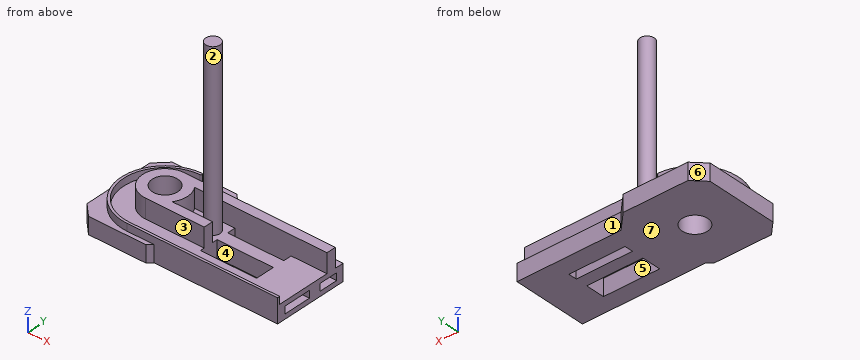
from build123d import *

# Parameters (mm, degrees)
SKETCH1_R               = 5.35
BOSS_EXTRUDE2_DEPTH     = 7
BOSS_EXTRUDE3_START     = 8
SKETCH3_R               = 5.35
BOSS_EXTRUDE3_DEPTH     = 8
BOSS_EXTRUDE4_DEPTH     = 3
CHAMFER1_SIZE           = 10
CHAMFER2_SIZE           = 5
CUT_EXTRUDE1_DEPTH      = 67.560662475
CUT_EXTRUDE1_DEPTH_BACK = 67.560662475
SKETCH5_W               = 23.474956737
SKETCH5_H               = 3.5
SKETCH5_H_2             = 8
CHAMFER3_SIZE           = 7
SKETCH6_W               = 3
SKETCH6_H               = 8.094956055
SKETCH6_H_2             = 11.655043945
CUT_EXTRUDE2_DEPTH      = 5
CUT_EXTRUDE3_REACH      = 87.249
SKETCH7_W               = 8
SKETCH7_H               = 4
SKETCH8_R               = 3
BOSS_EXTRUDE5_DEPTH     = 72
FILLET1_R               = 0.5


# Some blends are built 0.0001 mm under size
with BuildPart() as part:
    # Sketch1 → Boss-Extrude2 (new body)
    with BuildSketch(Plane.XY):
        Polygon((-19.503784034, -20), (19.503784034, -20), (19.503784034, -18.25), (62.978740771, -18.25), (62.978740771, 13), (19.503784034, 13), (19.503784034, 20), (-19.503784034, 20), align=None)
        Circle(SKETCH1_R, mode=Mode.SUBTRACT)
    extrude(amount=-BOSS_EXTRUDE2_DEPTH)

    # Sketch3 → Boss-Extrude3 (add)
    with BuildSketch(Plane.XY.offset(BOSS_EXTRUDE3_START)):
        with BuildLine():
            Line((7.668115805, 5.35), (62.978740771, 5.35))
            Line((62.978740771, 5.35), (62.978740771, 9.35))
            Line((62.978740771, 9.35), (0, 9.35))
            ThreePointArc((0, 9.35), (-9.35, 0), (0, -9.35))
            Line((0, -9.35), (62.978740771, -9.35))
            Line((62.978740771, -9.35), (62.978740771, -5.35))
            Line((62.978740771, -5.35), (7.668115805, -5.35))
            ThreePointArc((7.668115805, -5.35), (9.35, 0), (7.668115805, 5.35))
        make_face()
        Circle(SKETCH3_R, mode=Mode.SUBTRACT)
    extrude(amount=-BOSS_EXTRUDE3_DEPTH)

    # Sketch4 → Boss-Extrude4 (add)
    with BuildSketch(Plane.XY):
        with BuildLine():
            Line((0, -18.25), (62.978740771, -18.25))
            Line((62.978740771, -18.25), (62.978740771, -17.25))
            Line((62.978740771, -17.25), (8.306623863, -17.25))
            Line((8.306623863, -17.25), (0, -17.25))
            ThreePointArc((0, -17.25), (-17.25, 0), (0, 17.25))
            Line((0, 17.25), (0, 18.25))
            ThreePointArc((0, 18.25), (-18.25, 0), (0, -18.25))
        make_face()
    extrude(amount=BOSS_EXTRUDE4_DEPTH)

    # Chamfer1
    # the kernel refuses this chamfer: 10 mm, written as the material it takes off along each edge
    with BuildSketch(Plane(origin=(19.503784034, -20, 25.71682988), x_dir=(-0.9996219169112968, -0.027495876610586317, 0), z_dir=(0, 0, -1))) as chamfer1_piece_1_section:
        Polygon((CHAMFER1_SIZE * 0.999621916911, CHAMFER1_SIZE * 0.0274958766106), (-CHAMFER1_SIZE * 0.0274958766106, CHAMFER1_SIZE * 0.999621916911), (0, 0), align=None)
    chamfer1_piece_1 = extrude(amount=58.433659759, mode=Mode.PRIVATE)
    chamfer1_piece_1 = split(chamfer1_piece_1, bisect_by=Plane(origin=(14.814200223, -18.25, -3.5), z_dir=(0, -1, 0)), keep=Keep.TOP, mode=Mode.PRIVATE)
    add(chamfer1_piece_1, mode=Mode.SUBTRACT)

    # Chamfer2
    chamfer2_edges = [part.edges().sort_by_distance(p)[0] for p in [
        (-19.503784034, -20, -3.5),
        (-19.503784034, 20, -3.5),
    ]]
    chamfer(chamfer2_edges, length=CHAMFER2_SIZE)

    # Sketch5 → Cut-Extrude1 (cut, two sides: drawn at the far end of the back side and taken through both)
    with BuildSketch(Plane.XY.offset(-CUT_EXTRUDE1_DEPTH_BACK)):
        with Locations((36.241262403, 3.6)):
            Rectangle(SKETCH5_W, SKETCH5_H)
        with Locations((36.241262403, -7.15)):
            Rectangle(SKETCH5_W, SKETCH5_H_2)
    extrude(amount=CUT_EXTRUDE1_DEPTH + CUT_EXTRUDE1_DEPTH_BACK, mode=Mode.SUBTRACT)

    # Chamfer3
    chamfer3_edges = [part.edges().sort_by_distance(p)[0] for p in [
        (19.503784034, 20, -3.5),
    ]]
    chamfer(chamfer3_edges, length=CHAMFER3_SIZE - 0.0001)  # a hair under: the kernel refuses the full size

    # Sketch6 → Cut-Extrude2 (cut)
    with BuildSketch(Plane(origin=(62.978740771, 0, 0), x_dir=(0, 0, -1), z_dir=(1, 0, 0))):
        with Locations((3.5, 5.952521972)):
            Rectangle(SKETCH6_W, SKETCH6_H)
        with Locations((3.5, -8.922478028)):
            Rectangle(SKETCH6_W, SKETCH6_H_2)
    extrude(amount=-CUT_EXTRUDE2_DEPTH, mode=Mode.SUBTRACT)

    # Sketch7 → Cut-Extrude3 (cut, up to next)
    with BuildSketch(Plane(origin=(62.978740771, 0, 0), x_dir=(0, 0, -1), z_dir=(1, 0, 0)), mode=Mode.PRIVATE) as cut_extrude3_sk1:
        with Locations((-4, -7.35)):
            Rectangle(SKETCH7_W, SKETCH7_H)
    cut_extrude3_tool1 = extrude(cut_extrude3_sk1.sketch, amount=-CUT_EXTRUDE3_REACH, mode=Mode.PRIVATE) & part.part
    add(cut_extrude3_tool1.solids().sort_by_distance((62.978741, -7.35, 4))[0], mode=Mode.SUBTRACT)

    # Sketch8 → Boss-Extrude5 (add)
    with BuildSketch(Plane.XY):
        with Locations((20.003784034, 0)):
            Circle(SKETCH8_R)
    extrude(amount=BOSS_EXTRUDE5_DEPTH)

    # Fillet1
    fillet1_edges = [part.edges().sort_by_distance(p)[0] for p in [
        (0, 18.25, 1.5),
        (0, 17.25, 1.5),
    ]]
    fillet(fillet1_edges, radius=FILLET1_R - 0.0001)  # a hair under: the kernel refuses the full size


solid = part.part
For this review, take the finished solid that the model builds, in its own axes (mm). Face numbers are marked on the shaded views. A direction names the side the tool comes from. Give positions to 0.01 mm unless a question says otherwise; leave off trailing zeros. Loops run counter-clockwise (first coordinate to the right, second up) from the corner with the lowest first, then second, coordinate; pieces in that order, holes last.
Item 1: Tool access review of the marked faces 1, 2, 3 and 4: name each direction out of +Z, -Z, +X, -X, +Y, -Y from which nothing blocks a thin tool from reaching the whole face with its end or side.
Item 2: Take a section at B-B, the plane x = -3.5. State the section outline as (y, z) points, and give its area (3 significant figures).
Item 3: For line 1 along Y through (x, z) = (0, -1); line 2 along Z through (x, y) = (56, 8); line 3 along Z through (x, y) = (8, 11), list the stretches that pass through material, from the lowest coordinate up.
Item 4: Take a section at C-C, the plane x = 27. State the section outline as (y, z) points.
Item 5: Take a section at A-A, the plane y = 0. State the section outline as (x, z) points.
Item 6: Draft analysis for pull direction X (two halves, no side actions). For the marked faces 5, 6 and 7, state which applies: +X half, -X half, draft (parallel to the pull), parting line (faces both ways), or undercut.
Item 7: Take a section at D-D, the plane x = 51. State the section outline as (y, z) points, and give its area (3 significant figures).
Item 8: Insertion check: pin 1 (5.5 mm diameter, centred on x = 38.5, y = -1.5, fed in from +Z); pin 2 (17 mm diameter, centred on x = 0, y = 0, fed in from +Z); pin 3 (3.5 mm diameter, centred on x = 60, z = -3, fed in from -Y). Each pin has a flat end and moves straight along its axis. Give the tip position at first contact, or say it passes through.
Calculated:
1. face 1: +Z, -Z, +X, +Y
1. face 2: +Z
1. face 3: +Z, +X
1. face 4: +Z, -Z
2. outline: (-20, -7) - (-4.05, -7) - (-4.05, 8) - (-8.67, 8) - (-8.67, 0) - (-16.89, 0) - (-16.89, 3) - (-17.91, 3) - (-17.91, 0) - (-20, 0) - close; (4.05, -7) - (20, -7) - (20, 0) - (17.91, 0) - (17.91, 3) - (16.89, 3) - (16.89, 0) - (8.67, 0) - (8.67, 8) - (4.05, 8) - close
2. area: 303 mm2
3. line 1: y = -20 to -5.35, 5.35 to 20
3. line 2: z = -7 to 8
3. line 3: z = -7 to 0
4. outline: (-18.25, -7) - (-11.15, -7) - (-11.15, 0) - (-17.25, 0) - (-17.25, 3) - (-18.25, 3) - close; (-3.15, -7) - (1.85, -7) - (1.85, 0) - (-3.15, 0) - close; (5.35, -7) - (13, -7) - (13, 0) - (9.35, 0) - (9.35, 8) - (5.35, 8) - close
5. outline: (-19.5, -7) - (-5.35, -7) - (-5.35, 8) - (-9.35, 8) - (-9.35, 0) - (-17.25, 0) - (-17.25, 3) - (-18.25, 3) - (-18.25, 0) - (-19.5, 0) - close; (5.35, -7) - (62.98, -7) - (62.98, 0) - (23, 0) - (23, 72) - (17, 72) - (17, 0) - (9.35, 0) - (9.35, 8) - (5.35, 8) - close
6. face 5: undercut
6. face 6: -X half
6. face 7: draft
7. outline: (-18.25, -7) - (13, -7) - (13, 0) - (9.35, 0) - (9.35, 8) - (5.35, 8) - (5.35, 0) - (-17.25, 0) - (-17.25, 3) - (-18.25, 3) - close
7. area: 254 mm2
8. pin 1: stops at z = 0
8. pin 2: stops at z = 8
8. pin 3: stops at y = -18.25
